Could you check a few things on this drawing? It's one solid part, dimensions in mm from its lowest x, y, z. A direction names the side the tool comes from. Coordinates: 2 decimals unless noted, no trailing zeros. Write each loop counter-clockwise with the first axis right and the second up, starting at its lowest first coordinate (ties: lowest second). Pieces come first, ordered by that corner, then holes. Notation, with made-up numbers: M 68.5,48 L 126.5,48 A25 cw 126.5,74 Z; hole C 52,-10 d6. An arc over 180 degrees is marked long. Use a Markdown table: item, result.
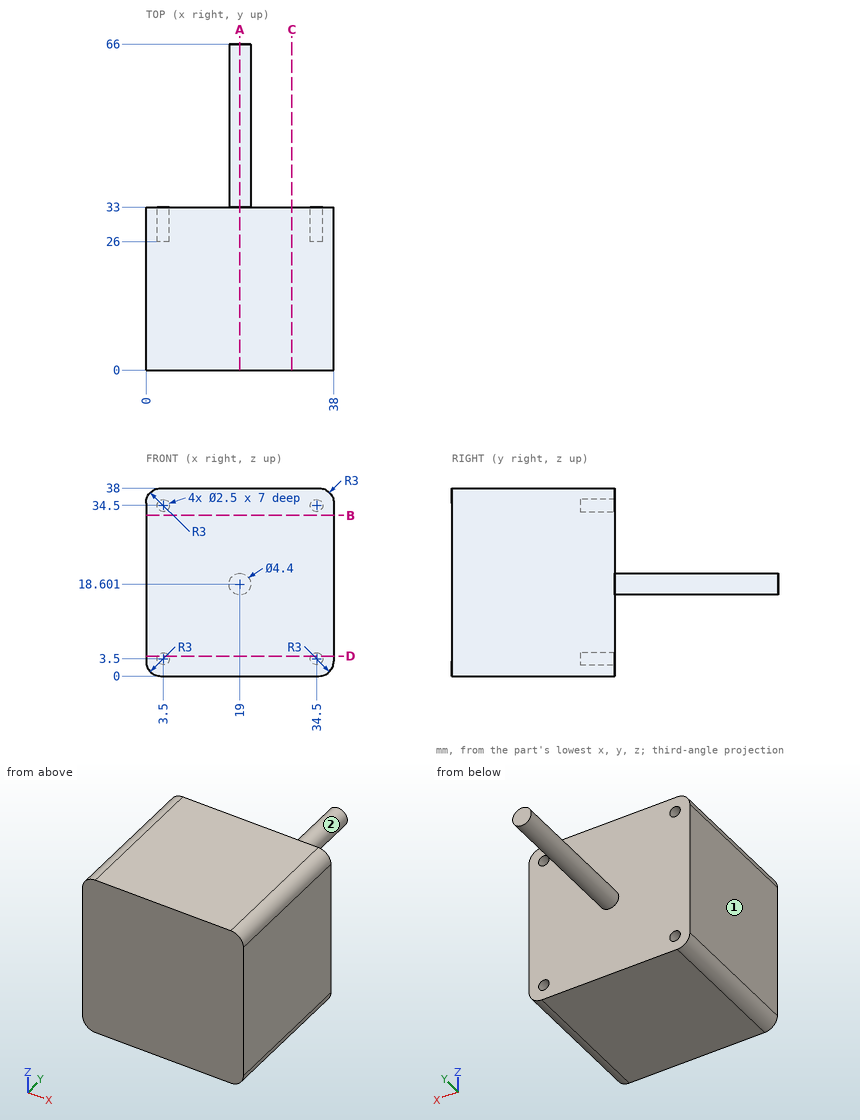
1. Will these pins go through, and if not, where does the flat tip stop? pin 1 Ø1 at (y, z) = (32, 10.5) entering from -X; pin 2 Ø3 at (x, z) = (34.5, 3.5) entering from +Y; pin 3 Ø12 at (x, y) = (15.5, 54.5) entering from +Z; pin 4 Ø0.7 at (x, z) = (3, 3.5) entering from +Y.
Answers follow:
| item | result |
|---|---|
| pin 1 | stops at x = 0 |
| pin 2 | stops at y = 33 |
| pin 3 | stops at z = 20.8 |
| pin 4 | stops at y = 26 |
2. Suppose I cut it at D-D on z = 4. Write out the boundary of the cut face in (x, y), and give its area (3 significant figures).
Answers follow:
| item | result |
|---|---|
| outline | M 0,0 L 38,0 L 38,33 L 35.65,33 L 35.65,26 L 33.35,26 L 33.35,33 L 4.65,33 L 4.65,26 L 2.35,26 L 2.35,33 L 0,33 Z |
| area | 1,220 mm2 |
3. Which directions (+Z, -Z, +X, -X, +Y, -Y) give clear straight access to the entire face, cutting with the end or side of a thin tool? Please do the marked faces 1 and 2.
Answers follow:
| item | result |
|---|---|
| face 1 | +Z, -Z, -X, +Y, -Y |
| face 2 | +Y |
4. Suppose I cut it at C-C on x = 29.5. Write out the boundary of the cut face in (y, z), and give its area (3 significant figures).
Answers follow:
| item | result |
|---|---|
| outline | M 0,0 L 33,0 L 33,38 L 0,38 Z |
| area | 1,250 mm2 |
5. I need wall thicknesses on probe 1 along X at (y, z) = (29.5, 3.5); probe 2 along X at (y, z) = (30, 34). Which ranges of each line are inside material? Lowest first, please.
Answers follow:
| item | result |
|---|---|
| probe 1 | x = 0 to 2.25, 4.75 to 33.25, 35.75 to 38 |
| probe 2 | x = 0 to 2.35, 4.65 to 33.35, 35.65 to 38 |
6. Suppose I cut it at B-B on z = 32.5. Write out the boundary of the cut face in (x, y).
Answers follow:
| item | result |
|---|---|
| outline | M 0,0 L 38,0 L 38,33 L 0,33 Z |
7. Suppose I cut it at A-A on x = 19. Write out the boundary of the cut face in (y, z), and give its area (3 significant figures).
Answers follow:
| item | result |
|---|---|
| outline | M 0,0 L 33,0 L 33,16.4 L 66,16.4 L 66,20.8 L 33,20.8 L 33,38 L 0,38 Z |
| area | 1,400 mm2 |
